Can you work these out from the drawing? Everything is in mm from the part's minimum corner. Coordinates: 2 decimals unless noted, no trailing zeros. Write each loop counter-clockwise with the first axis right and the second up, starting at its lowest first coordinate (ties: lowest second). Pieces come first, ordered by that corner, then holes. Notation, with made-up numbers: (37, -32) -> (69, -32) arc R34 cw to (69, 0) -> close; hole circle Ø4 at (-8.5, 68). An arc over 180 degrees is marked (long way). Use CSV: the item, a comma, the result in double quotes. Start each with the question number.
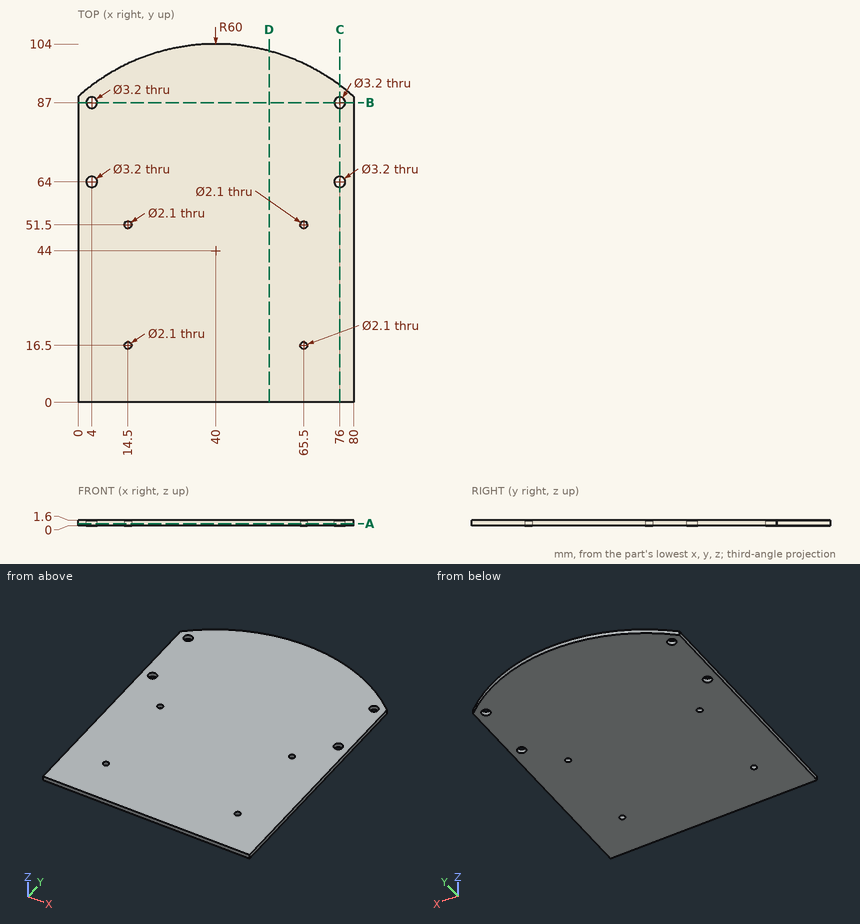
Item 1: I want a section at C-C on x = 76. Please give me the cut outline in (y, z), then the cut area to 3 significant figures.
Item 2: If I drill on line 1 along X through (y, z) = (16.5, 1.15); line 2 along X through (y, z) = (87, 1.2); line 3 along Y through (x, z) = (14.5, 1.25), over which ranges is the centre line in solid material (lowest first)?
Item 3: I want a section at A-A on z = 0.65. Count the separate pieces of the cut face and the enclosed holes in it, then the cut area to 3 significant figures.
Item 4: I want a section at D-D on x = 55.5. Please give me the cut outline in (y, z).
Item 5: I want a section at B-B on y = 87. Please give me the cut outline in (x, z), then the cut area to 3 significant figures.
Geometry says:
1,outline,"(0, 0) -> (62.4, 0) -> (62.4, 1.6) -> (0, 1.6) -> close; (65.6, 0) -> (85.4, 0) -> (85.4, 1.6) -> (65.6, 1.6) -> close; (88.6, 0) -> (92, 0) -> (92, 1.6) -> (88.6, 1.6) -> close"
1,area,"137 mm2"
2,line 1,"0 to 13.45, 15.55 to 64.45, 66.55 to 80"
2,line 2,"0 to 2.4, 5.6 to 74.4, 77.6 to 80"
2,line 3,"0 to 15.45, 17.55 to 50.45, 52.55 to 98.31"
3,separate pieces,"1"
3,enclosed holes,"8"
3,area,"7,890 mm2"
4,outline,"(0, 0) -> (101.96, 0) -> (101.96, 1.6) -> (0, 1.6) -> close"
5,outline,"(0, 0) -> (2.4, 0) -> (2.4, 1.6) -> (0, 1.6) -> close; (5.6, 0) -> (74.4, 0) -> (74.4, 1.6) -> (5.6, 1.6) -> close; (77.6, 0) -> (80, 0) -> (80, 1.6) -> (77.6, 1.6) -> close"
5,area,"118 mm2"
